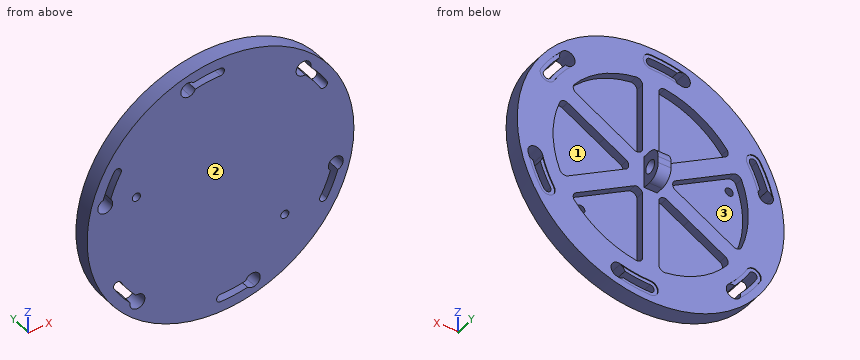
from build123d import *

# Parameters (mm, degrees)
SKETCH1_R           = 82
BOSS_EXTRUDE1_DEPTH = 10
BOSS_EXTRUDE3_DEPTH = 9.525
CIRPATTERN1_COUNT   = 6
CUT_EXTRUDE1_DEPTH  = 5
SKETCH3_R           = 2.5
CUT_EXTRUDE2_DEPTH  = 5
SKETCH3_3_R         = 2.5
CUT_EXTRUDE3_DEPTH  = 5
SKETCH5_W           = 7.911182114
SKETCH5_H           = 19.959178222
BOSS_EXTRUDE5_DEPTH = 12.5
FILLET2_R           = 8
SKETCH7_R           = 4
CUT_EXTRUDE4_DEPTH  = 8.5


with BuildPart() as part:
    # Sketch1 → Boss-Extrude1 (new body)
    with BuildSketch(Plane(origin=(0, 0, 0), x_dir=(1, 0, 0), z_dir=(0, 1, 0))):
        Circle(SKETCH1_R)
        with BuildLine():
            ThreePointArc((0, -68.539794907), (4.585205093, -73.125), (0, -77.710205093))
            ThreePointArc((0, -77.710205093), (-10.627709007, -76.980047914), (-21.05570427, -74.803297343))
            ThreePointArc((-21.05570427, -74.803297343), (-24.227021824, -69.147242492), (-18.570966974, -65.975924939))
            ThreePointArc((-18.570966974, -65.975924939), (-9.373556469, -67.895801969), (0, -68.539794907))
        make_face(mode=Mode.SUBTRACT)
        with BuildLine():
            ThreePointArc((-59.357203559, -34.269897453), (-61.035505105, -40.533404092), (-67.299011744, -38.855102547))
            ThreePointArc((-67.299011744, -38.855102547), (-71.980531582, -29.286157973), (-75.309407921, -19.166873879))
            ThreePointArc((-75.309407921, -19.166873879), (-71.996779512, -13.592404889), (-66.422310522, -16.905033297))
            ThreePointArc((-66.422310522, -16.905033297), (-63.48626755, -25.830162958), (-59.357203559, -34.269897453))
        make_face(mode=Mode.SUBTRACT)
        with BuildLine():
            ThreePointArc((59.357203559, -34.269897453), (65.620710198, -32.591595908), (67.299011744, -38.855102547))
            ThreePointArc((67.299011744, -38.855102547), (61.352822575, -47.693889942), (54.25370365, -55.636423464))
            ThreePointArc((54.25370365, -55.636423464), (47.769757688, -55.554837604), (47.851343548, -49.070891641))
            ThreePointArc((47.851343548, -49.070891641), (54.112711081, -42.065639011), (59.357203559, -34.269897453))
        make_face(mode=Mode.SUBTRACT)
        with BuildLine():
            ThreePointArc((-59.357203559, 34.269897453), (-65.620710198, 32.591595908), (-67.299011744, 38.855102547))
            ThreePointArc((-67.299011744, 38.855102547), (-61.352822575, 47.693889942), (-54.25370365, 55.636423464))
            ThreePointArc((-54.25370365, 55.636423464), (-47.769757688, 55.554837604), (-47.851343548, 49.070891641))
            ThreePointArc((-47.851343548, 49.070891641), (-54.112711081, 42.065639011), (-59.357203559, 34.269897453))
        make_face(mode=Mode.SUBTRACT)
        with BuildLine():
            ThreePointArc((59.357203559, 34.269897453), (61.035505105, 40.533404092), (67.299011744, 38.855102547))
            ThreePointArc((67.299011744, 38.855102547), (71.980531582, 29.286157973), (75.309407921, 19.166873879))
            ThreePointArc((75.309407921, 19.166873879), (71.996779512, 13.592404889), (66.422310522, 16.905033297))
            ThreePointArc((66.422310522, 16.905033297), (63.48626755, 25.830162958), (59.357203559, 34.269897453))
        make_face(mode=Mode.SUBTRACT)
        with BuildLine():
            ThreePointArc((0, 68.539794907), (-4.585205093, 73.125), (0, 77.710205093))
            ThreePointArc((0, 77.710205093), (10.627709007, 76.980047914), (21.05570427, 74.803297343))
            ThreePointArc((21.05570427, 74.803297343), (24.227021824, 69.147242492), (18.570966974, 65.975924939))
            ThreePointArc((18.570966974, 65.975924939), (9.373556469, 67.895801969), (0, 68.539794907))
        make_face(mode=Mode.SUBTRACT)
    extrude(amount=BOSS_EXTRUDE1_DEPTH)

    # Sketch1_4 → Boss-Extrude3 (add)
    with BuildSketch(Plane(origin=(0, 0, 0), x_dir=(1, 0, 0), z_dir=(0, 1, 0))):
        with BuildLine():
            ThreePointArc((-75.309407921, -19.166873879), (-71.980531582, -29.286157973), (-67.299011744, -38.855102547))
            ThreePointArc((-67.299011744, -38.855102547), (-61.035505105, -40.533404092), (-59.357203559, -34.269897453))
            ThreePointArc((-59.357203559, -34.269897453), (-63.48626755, -25.830162958), (-66.422310522, -16.905033297))
            ThreePointArc((-66.422310522, -16.905033297), (-66.418285743, -19.150940539), (-67.48132535, -21.129339471))
            ThreePointArc((-67.48132535, -21.129339471), (-64.751733563, -28.414631056), (-61.238335159, -35.355969289))
            ThreePointArc((-61.238335159, -35.355969289), (-62.121576941, -38.652272492), (-65.417880144, -37.769030711))
            ThreePointArc((-65.417880144, -37.769030711), (-69.197773577, -30.293016611), (-72.126599919, -22.444427093))
            ThreePointArc((-72.126599919, -22.444427093), (-74.155284422, -21.230290389), (-75.309407921, -19.166873879))
        make_face()
    boss_extrude3 = extrude(amount=BOSS_EXTRUDE3_DEPTH)

    # CirPattern1: Boss-Extrude3 ×6 about axis
    cirpattern1_axis = Axis((0, 0, 0), (0, 1, 0))
    for i in range(1, CIRPATTERN1_COUNT):
        add(boss_extrude3.rotate(cirpattern1_axis, i * 360 / CIRPATTERN1_COUNT))

    # Sketch2 → Cut-Extrude1 (cut)
    with BuildSketch(Plane(origin=(0, 10, 0), x_dir=(1, 0, 0), z_dir=(0, 1, 0))):
        with BuildLine():
            ThreePointArc((-55.779211114, 22.106098875), (-53.723615936, 23.879831653), (-51.015872171, 23.680524839))
            Line((-51.015872171, 23.680524839), (-28.480762114, 10.669872981))
            Line((-28.480762114, 10.669872981), (-14.620190528, 2.667468245))
            ThreePointArc((-14.620190528, 2.667468245), (-13.515289004, 0), (-14.620190528, -2.667468245))
            Line((-14.620190528, -2.667468245), (-28.480762114, -10.669872981))
            Line((-28.480762114, -10.669872981), (-51.015872171, -23.680524839))
            ThreePointArc((-51.015872171, -23.680524839), (-53.723615936, -23.879831653), (-55.779211114, -22.106098875))
            ThreePointArc((-55.779211114, -22.106098875), (-60, 0), (-55.779211114, 22.106098875))
        make_face()
        with BuildLine():
            ThreePointArc((-8.745162353, 59.359263266), (-6.181267118, 58.46593201), (-5, 56.021303716))
            Line((-5, 56.021303716), (-5, 30))
            Line((-5, 30), (-5, 13.995190528))
            ThreePointArc((-5, 13.995190528), (-6.757644502, 11.704583617), (-9.620190528, 11.327722283))
            Line((-9.620190528, 11.327722283), (-23.480762114, 19.330127019))
            Line((-23.480762114, 19.330127019), (-46.015872171, 32.340778877))
            ThreePointArc((-46.015872171, 32.340778877), (-47.542348818, 34.586100357), (-47.034048761, 37.253164391))
            ThreePointArc((-47.034048761, 37.253164391), (-30, 51.961524227), (-8.745162353, 59.359263266))
        make_face()
        with BuildLine():
            ThreePointArc((47.034048761, 37.253164391), (47.542348818, 34.586100357), (46.015872171, 32.340778877))
            Line((46.015872171, 32.340778877), (23.480762114, 19.330127019))
            Line((23.480762114, 19.330127019), (9.620190528, 11.327722283))
            ThreePointArc((9.620190528, 11.327722283), (6.757644502, 11.704583617), (5, 13.995190528))
            Line((5, 13.995190528), (5, 30))
            Line((5, 30), (5, 56.021303716))
            ThreePointArc((5, 56.021303716), (6.181267118, 58.46593201), (8.745162353, 59.359263266))
            ThreePointArc((8.745162353, 59.359263266), (30, 51.961524227), (47.034048761, 37.253164391))
        make_face()
        with BuildLine():
            ThreePointArc((55.779211114, -22.106098875), (53.723615936, -23.879831653), (51.015872171, -23.680524839))
            Line((51.015872171, -23.680524839), (28.480762114, -10.669872981))
            Line((28.480762114, -10.669872981), (14.620190528, -2.667468245))
            ThreePointArc((14.620190528, -2.667468245), (13.515289004, 0), (14.620190528, 2.667468245))
            Line((14.620190528, 2.667468245), (28.480762114, 10.669872981))
            Line((28.480762114, 10.669872981), (51.015872171, 23.680524839))
            ThreePointArc((51.015872171, 23.680524839), (53.723615936, 23.879831653), (55.779211114, 22.106098875))
            ThreePointArc((55.779211114, 22.106098875), (60, 0), (55.779211114, -22.106098875))
        make_face()
        with BuildLine():
            ThreePointArc((8.745162353, -59.359263266), (6.181267118, -58.46593201), (5, -56.021303716))
            Line((5, -56.021303716), (5, -30))
            Line((5, -30), (5, -13.995190528))
            ThreePointArc((5, -13.995190528), (6.757644502, -11.704583617), (9.620190528, -11.327722283))
            Line((9.620190528, -11.327722283), (23.480762114, -19.330127019))
            Line((23.480762114, -19.330127019), (46.015872171, -32.340778877))
            ThreePointArc((46.015872171, -32.340778877), (47.542348818, -34.586100357), (47.034048761, -37.253164391))
            ThreePointArc((47.034048761, -37.253164391), (30, -51.961524227), (8.745162353, -59.359263266))
        make_face()
        with BuildLine():
            ThreePointArc((-5, -56.021303716), (-6.181267118, -58.46593201), (-8.745162353, -59.359263266))
            ThreePointArc((-8.745162353, -59.359263266), (-30, -51.961524227), (-47.034048761, -37.253164391))
            ThreePointArc((-47.034048761, -37.253164391), (-47.542348818, -34.586100357), (-46.015872171, -32.340778877))
            Line((-46.015872171, -32.340778877), (-23.480762114, -19.330127019))
            Line((-23.480762114, -19.330127019), (-9.620190528, -11.327722283))
            ThreePointArc((-9.620190528, -11.327722283), (-6.757644502, -11.704583617), (-5, -13.995190528))
            Line((-5, -13.995190528), (-5, -30))
            Line((-5, -30), (-5, -56.021303716))
        make_face()
    extrude(amount=-CUT_EXTRUDE1_DEPTH, mode=Mode.SUBTRACT)

    # Sketch3 → Cut-Extrude2 (cut)
    with BuildSketch(Plane.XZ):
        with Locations((-51.685176347, 15.403969857)):
            Circle(SKETCH3_R)
    extrude(amount=-CUT_EXTRUDE2_DEPTH, mode=Mode.SUBTRACT)

    # Sketch3_3 → Cut-Extrude3 (cut)
    with BuildSketch(Plane.XZ):
        with Locations((39.514507533, -36.782411469)):
            Circle(SKETCH3_3_R)
    extrude(amount=-CUT_EXTRUDE3_DEPTH, mode=Mode.SUBTRACT)

    # Sketch5 → Boss-Extrude5 (add)
    with BuildSketch(Plane(origin=(0, 10, 0), x_dir=(1, 0, 0), z_dir=(0, 1, 0))):
        Rectangle(SKETCH5_W, SKETCH5_H)
    extrude(amount=BOSS_EXTRUDE5_DEPTH)

    # Fillet2
    fillet2_edges = [part.edges().sort_by_distance(p)[0] for p in [
        (0, 22.5, 9.979589111),
        (0, 22.5, -9.979589111),
    ]]
    fillet(fillet2_edges, radius=FILLET2_R)

    # Sketch7 → Cut-Extrude4 (cut)
    with BuildSketch(Plane.ZY.offset(3.955591057)):
        with Locations((0, 15.342929393)):
            Circle(SKETCH7_R)
    extrude(amount=-CUT_EXTRUDE4_DEPTH, mode=Mode.SUBTRACT)


solid = part.part
Geometry check sheet. Reference: the model listing, model coordinates, mm. Face numbers are marked on the shaded views. Round coordinates to 2 decimals unless told otherwise and drop trailing zeros. Loops run counter-clockwise (first coordinate to the right, second up) from the corner with the lowest first, then second, coordinate; pieces in that order, holes last. Notation, with made-up numbers: (19, 66) -> (41, 66) arc R26 cw to (41, 87) -> close; hole circle Ø1 at (-25, 34). An arc over 180 degrees is marked (long way). Answer as a JSON object with one key per item and string values. Group by question number.
Item 1: Thickness scan on line 1 along Y through (x, z) = (2, 0); line 2 along Z through (x, y) = (24, 9.25); line 3 along Z through (x, y) = (-26.5, 8.75). Record the ranges inside material, lowest first.
Item 2: Depth check by flat-ended pin: pin 1 Ø2 at (x, y) = (-0.5, 19.5) entering from +Z; pin 2 Ø1 at (x, y) = (-50, 6.5) entering from +Z; pin 3 Ø5 at (x, z) = (-22.5, 56.5) entering from +Y. Enter the tip coordinate at first touch or a pass-through.
Item 3: Release check for a two-part mould opening along X. For the marked faces 1, 2 and 3 record: pulls with the +X half, pulls with the -X half, needs draft (parallel to the pull), parting line crosses it, or undercut.
Item 4: Cross-section at A-A, the plane z = 0. Record the cut outline in (x, y), plus the area to 3 significant figures.
Determined:
{
 "1": {"line 1": "y = 0 to 11.34, 19.34 to 22.5", "line 2": "z = -78.41 to -72.26, -68.52 to -54.99, -19.63 to -8.08, 8.08 to 19.63, 54.99 to 78.41", "line 3": "z = -77.6 to -53.83, -21.07 to -9.53, 9.53 to 21.07, 53.83 to 77.6"},
 "2": {"pin 1": "stops at z = 8.91", "pin 2": "stops at z = 65.37", "pin 3": "stops at y = 10"},
 "3": {"face 1": "undercut", "face 2": "needs draft", "face 3": "undercut"},
 "4": {"outline": "(-82, 0) -> (82, 0) -> (82, 10) -> (60, 10) -> (60, 5) -> (13.52, 5) -> (13.52, 10) -> (3.96, 10) -> (3.96, 11.34) -> (-3.96, 11.34) -> (-3.96, 10) -> (-13.52, 10) -> (-13.52, 5) -> (-60, 5) -> (-60, 10) -> (-82, 10) -> close; (-3.96, 19.34) -> (3.96, 19.34) -> (3.96, 22.5) -> (-3.96, 22.5) -> close", "area": "1,210 mm²"}
}
